from build123d import *

# Parameters (mm, degrees)
CUT_EXTRUDE1_DEPTH = 3.175
FILLET1_R          = 0.79375
CHAMFER1_SIZE      = 0.254


with BuildPart() as part:
    # Sketch1 → Revolve1 (revolve)
    with BuildSketch(Plane.XY):
        Polygon((3.175, 0), (6.35, 0), (6.35, 6.35), (2.9845, 6.35), (2.9845, 47.625), (1.5875, 47.625), (1.5875, 3.175), (3.175, 3.175), align=None)
    revolve(axis=Axis((0, 5.569325848, 0), (0, -1, 0)))

    # Sketch2 → Cut-Extrude1 (cut)
    with BuildSketch(Plane.XZ):
        Polygon((1.833087105, 3.175), (-1.833087105, 3.175), (-3.666174209, 0), (-1.833087105, -3.175), (1.833087105, -3.175), (3.666174209, 0), align=None)
    extrude(amount=-CUT_EXTRUDE1_DEPTH, mode=Mode.SUBTRACT)

    # Fillet1
    fillet1_edges = [part.edges().sort_by_distance(p)[0] for p in [
        (0, 3.175, 3.175),
        (-2.749630657, 3.175, 1.5875),
        (-2.749630657, 3.175, -1.5875),
        (0, 3.175, -3.175),
        (2.749630657, 3.175, -1.5875),
        (2.749630657, 3.175, 1.5875),
        (-1.833087105, 1.5875, 3.175),
        (-3.666174209, 1.5875, 0),
        (-1.833087105, 1.5875, -3.175),
        (1.833087105, 1.5875, -3.175),
        (3.666174209, 1.5875, 0),
        (1.833087105, 1.5875, 3.175),
        (-2.9845, 6.35, 0),
    ]]
    fillet(fillet1_edges, radius=FILLET1_R)

    # Chamfer1
    chamfer1_edges = [part.edges().sort_by_distance(p)[0] for p in [
        (-1.5875, 3.175, 0),
        (0, 0, 3.175),
        (2.749630657, 0, 1.5875),
        (-1.5875, 47.625, 0),
        (2.749630657, 0, -1.5875),
        (0, 0, -3.175),
        (-2.9845, 47.625, 0),
        (-2.749630657, 0, -1.5875),
        (-2.749630657, 0, 1.5875),
        (-1.771690329, 0, 3.068657664),
        (1.771690329, 0, 3.068657664),
        (3.543380657, 0, 0),
        (1.771690329, 0, -3.068657664),
        (-1.771690329, 0, -3.068657664),
        (-3.543380657, 0, 0),
        (-6.35, 6.35, 0),
        (-6.35, 0, 0),
    ]]
    chamfer(chamfer1_edges, length=CHAMFER1_SIZE)


solid = part.part
Geometry check sheet. Reference: the model listing, model coordinates, mm. A direction names the side the tool comes from. Give positions to 0.01 mm unless a question says otherwise; leave off trailing zeros. Write each loop counter-clockwise with the first axis right and the second up, starting at its lowest first coordinate (ties: lowest second). Pieces come first, ordered by that corner, then holes.
1) Go/stop test with flat-tipped pins: pin 1 Ø0.6 at (x, y) = (-0.5, 1) entering from -Z; pin 2 Ø1.9 at (x, z) = (0, 0) entering from -Y; pin 3 Ø4 at (x, z) = (1.5, -5) entering from -Y; pin 4 Ø5 at (y, z) = (34, -4.5) entering from -X. Record where each tip stops, or that it passes through.
Values follow:
pin 1: stops at z = -6.35
pin 2: passes through
pin 3: stops at y = 0
pin 4: stops at x = -2.22
2) Thickness scan on line 1 (Z direction, x = 0, y = 36); line 2 (Y direction, x = 4.5, z = 3); line 3 (X direction, y = 16.5, z = -0.5). Record the ranges inside material, lowest first.
Values follow:
line 1: z = -2.98 to -1.59, 1.59 to 2.98
line 2: y = 0 to 6.35
line 3: x = -2.94 to -1.51, 1.51 to 2.94
3) Cross-section at B-B (y = 9). Record the boundary of the cut face in (x, z) (1 decimal), plus the area to 3 significant figures.
Values follow:
outline: circle Ø6 at (0, 0); hole circle Ø3.2 at (0, 0)
area: 20.1 mm2
4) Release check for a two-part mould opening along Z. For faces 1 (the face through (-3, 0, -3)), 2 (the face through (-2.87, 0.13, 1.63)), 3 (the face through (-0.647, 27.539, -2.914)), 4 (the face through (2, 3.175, 0)) record: released by +Z, released by -Z, zero draft, split by the parting line, or undercut.
Values follow:
face 1: zero draft
face 2: undercut
face 3: split by the parting line
face 4: undercut
5) Set-up check for faces 5 (the face through (-2.848, 0.129, -1.667)), 6 (the face through (1, 47.625, -2)): record each of +Z, -Z, +X, -X, +Y, -Y from which the full face is reachable in a straight line by a thin tool's end or side.
Values follow:
face 5: -Y
face 6: +Z, -Z, +X, -X, +Y
